Check sheet for the modelled part. Datum: model origin and axes. Units: mm. A direction names the side the tool comes from. Round coordinates to 2 decimals unless told otherwise and drop trailing zeros. Write each loop counter-clockwise with the first axis right and the second up, starting at its lowest first coordinate (ties: lowest second). Pieces come first, ordered by that corner, then holes. Notation, with made-up numbers: (-1.75, 8.25) - (23.25, 8.25) arc R18 cw to (23.25, 41.25) - close; hole circle Ø3 at (-2.75, 63.25). An arc over 180 degrees is marked (long way). Answer as a JSON object with one key per item and string values. Group by question number.
Item 1: Set-up check for faces 1 (the flat face through (19, -62.454, 12)), 2 (the flat face through (19.05, -50, 27)): record each of +Z, -Z, +X, -X, +Y, -Y from which the full face is reachable in a straight line by a thin tool's end or side.
Item 2: Sectioned sample at B-B on x = 40. Record the boundary of the cut face in (y, z).
Item 3: Sectioned sample at C-C on z = 20.5. Record the boundary of the cut face in (x, y), plus the area to 3 significant figures.
Item 4: Thickness scan on line 1 (X direction, y = -33, z = 34); line 2 (Z direction, x = 19.5, y = -59.5); line 3 (Z direction, x = 36, y = -56.5). Record the ranges inside material, lowest first.
Item 5: Gauge pin test, flat ends, axial feed: P1, Ø10, axis at x = 32, z = 26, coming from the -Y side; P2, Ø5, axis at x = 45, y = -43, coming from the +Z side; P3, Ø3, axis at x = 43, y = -49.5, coming from the +Z side. Record the tip position at first contact, or that the pin passes through.
Item 6: Sectioned sample at A-A on y = -56. Record the boundary of the cut face in (x, z), plus the area to 3 significant figures.
```python
from build123d import *

# Parameters (mm, degrees)
F0_W     = 38.1
F0_H     = 31.75
F1_DEPTH = 25.4
F3_DEPTH = 25.4
F4_DEPTH = 6.35


with BuildPart() as f1:
    # F0 (on Right) → F1 (new body)
    with BuildSketch(Plane.YZ):
        with Locations((-43.4044748545, 19.3160282822)):
            Rectangle(F0_W, F0_H)
    extrude(amount=F1_DEPTH)

    # F2 (on face) → F3 (join)
    with BuildSketch(Plane.YZ.offset(25.4)):
        Polygon((-24.3544748545, 35.1910282822), (-30.5013419502, 35.1910282822), (-62.4544748545, 14.43994885), (-62.4544748545, 3.4410282822), (-24.3544748545, 3.4410282822), align=None)
    extrude(amount=F3_DEPTH)

    # F4 (cut): a face of the model
    f4_faces = [f1.faces().sort_by_distance(p)[0] for p in [
        (25.4, -51.8034305531, 28.2740018048),
    ]]
    extrude(f4_faces, amount=-F4_DEPTH, mode=Mode.SUBTRACT)


solid = f1.part
```
Completed:
{
 "1": {"face 1": "+Z, -Z, +X, -X, -Y", "face 2": "+Z, +X, -Y"},
 "2": {"outline": "(-62.45, 3.44) - (-24.35, 3.44) - (-24.35, 35.19) - (-30.5, 35.19) - (-62.45, 14.44) - close"},
 "3": {"outline": "(0, -62.45) - (19.05, -62.45) - (19.05, -53.12) - (50.8, -53.12) - (50.8, -24.35) - (0, -24.35) - close", "area": "1,640 mm²"},
 "4": {"line 1": "0 to 19.05", "line 2": "3.44 to 16.36", "line 3": "3.44 to 18.31"},
 "5": {"P1": "y = -52.35", "P2": "z = 28.7", "P3": "z = 23.83"},
 "6": {"outline": "(0, 3.44) - (50.8, 3.44) - (50.8, 18.63) - (19.05, 18.63) - (19.05, 35.19) - (0, 35.19) - close", "area": "1,090 mm²"}
}
